Autodesk Inventor part; units mm, degrees
ref_plane "YZ Plane" through (0, 0, 0) normal (1, 0, 0) x (0, 1, 0)
ref_plane "XZ Plane" through (0, 0, 0) normal (0, 1, 0) x (-1, 0, 0)
ref_plane "XY Plane" through (0, 0, 0) normal (0, 0, 1) x (1, 0, 0)
sketch "Sketch1" plane through (0, 0, 0) normal (0, 1, 0) x (-1, 0, 0)
  line L0 (84.709, 4.7625) -> (-84.709, 4.7625)
  line L1 (-84.709, 4.7625) -> (-84.709, -4.7625)
  line L2 (-84.709, -4.7625) -> (84.709, -4.7625)
  line L3 (84.709, -4.7625) -> (84.709, 4.7625)
  line L4 (4.7625, 62.5475) -> (-4.7625, 62.5475)
  line L5 (-4.7625, 62.5475) -> (-4.7625, -91.4781)
  line L6 (-4.7625, -91.4781) -> (4.7625, -91.4781)
  line L7 (4.7625, -91.4781) -> (4.7625, 62.5475)
  point P0 (0, 0)
  point P1 (0, -4.7625)
  point P2 (84.709, 0)
  point P3 (4.7625, -14.4653)
  point P4 (0, 62.5475)
  dimension "d0" = 9.525
  dimension "d1" = 169.418
  dimension "d2" = 154.0256
  dimension "d6" = 57.785
extrude "Extrusion1" add sketch "Sketch1" along normal blind 6.35
sketch "Sketch2" plane through (0, 6.35, 0) normal (0, 1, 0) x (1, 0, 0)
  line L0 (4.7625, 91.4781) -> (-4.7625, 91.4781)
  line L1 (84.709, -4.7625) -> (84.709, 4.7625)
  line L2 (-4.7625, -62.5475) -> (4.7625, -62.5475)
  line L3 (-84.709, 4.7625) -> (-84.709, -4.7625)
  point P0 (0, 0)
  point P1 (0, 86.7791)
  point P2 (0, -57.8485)
  point P3 (-80.01, 0)
  point P4 (80.01, 0)
  dimension "d7" = 4.699
  dimension "d8" = 4.699
  dimension "d9" = 4.699
  dimension "d10" = 4.699
hole "Hole1" at (0, 6.35, -86.7791) at (0, 6.35, 57.8485) at (-80.01, 6.35, 0) at (80.01, 6.35, 0) direction (0, -1, 0) diameter 3.302 end through all
fillet "Fillet1" radius 1.27 20 edges at (-44.7358, 6.35, 4.7625) (4.7625, 6.35, 33.655) (-4.7625, 6.35, 33.655) (44.7357, 6.35, 4.7625) (4.7625, 6.35, -48.1203) (-4.7625, 6.35, -48.1203) (-44.7357, 6.35, -4.7625) (44.7358, 6.35, -4.7625) (84.709, 3.175, 4.7625) (84.709, 3.175, -4.7625) (84.709, 6.35, 0) (4.7625, 3.175, 62.5475) (0, 6.35, 62.5475) (-4.7625, 3.175, 62.5475) (-84.709, 3.175, 4.7625) (-84.709, 6.35, 0) (4.7625, 3.175, -91.4781) (0, 6.35, -91.4781) (-4.7625, 3.175, -91.4781) (-84.709, 3.175, -4.7625)
fillet "Fillet2" radius 1.27 8 edges at (4.3905, 5.978, 4.3905) (4.7625, 2.54, 4.7625) (4.3905, 5.978, -4.3905) (4.7625, 2.54, -4.7625) (-4.3905, 5.978, -4.3905) (-4.7625, 2.54, -4.7625) (-4.3905, 5.978, 4.3905) (-4.7625, 2.54, 4.7625)
properties part number "BatteryCrossStrap"
Here's how the part is built. I have some questions about the finished solid (model axes, mm). A direction names the side the tool comes from. Round coordinates to 2 decimals unless told otherwise and drop trailing zeros. Write each loop counter-clockwise with the first axis right and the second up, starting at its lowest first coordinate (ties: lowest second). Pieces come first, ordered by that corner, then holes.
1. Suppose I cut it at C-C (z = 29). List the corners of the cut face in (x, y) for me, and give its area (3 significant figures).
2. Suppose I cut it at A-A (y = 3). List the corners of the cut face in (x, z) for me.
3. Will these pins go through, and if not, where does the flat tip stop? pin 1 Ø1.5 at (y, z) = (2, 25.5) entering from -X; pin 2 Ø3 at (x, y) = (-28.5, 2) entering from +Z; pin 3 Ø1.5 at (y, z) = (3, -28.5) entering from +X.
4. For faces 1 (the flat face through (-4.762, 3, -49)), 2 (the flat face through (44, 3, 4.762)), 3 (the flat face through (-4.762, 3, 33)), which set-ups out of +Z, -Z, +X, -X, +Y, -Y let a thin tool reach every point of the face, with its end or its side?
5. I need wall thicknesses on L1, parallel to X at y = 2, z = 0; L2, parallel to Z at x = -80.01, y = 4.5; L3, parallel to X at y = 4.75, z = 12. Which ranges of each line are inside material? Lowest first, please.
6. Suppose I cut it at B-B (x = -55.5). List the corners of the cut face in (y, z) for me.
Answer sheet:
1. outline: (-4.76, 0) - (4.76, 0) - (4.76, 5.08) arc R1.27 ccw to (3.49, 6.35) - (-3.49, 6.35) arc R1.27 ccw to (-4.76, 5.08) - close
1. area: 59.8 mm2
2. outline: (-84.71, -3.49) arc R1.27 ccw to (-83.44, -4.76) - (-6.03, -4.76) arc R1.27 cw to (-4.76, -6.03) - (-4.76, -90.21) arc R1.27 ccw to (-3.49, -91.48) - (3.49, -91.48) arc R1.27 ccw to (4.76, -90.21) - (4.76, -6.03) arc R1.27 cw to (6.03, -4.76) - (83.44, -4.76) arc R1.27 ccw to (84.71, -3.49) - (84.71, 3.49) arc R1.27 ccw to (83.44, 4.76) - (6.03, 4.76) arc R1.27 cw to (4.76, 6.03) - (4.76, 61.28) arc R1.27 ccw to (3.49, 62.55) - (-3.49, 62.55) arc R1.27 ccw to (-4.76, 61.28) - (-4.76, 6.03) arc R1.27 cw to (-6.03, 4.76) - (-83.44, 4.76) arc R1.27 ccw to (-84.71, 3.49) - close; hole circle Ø3.3 at (-80.01, 0); hole circle Ø3.3 at (0, -86.78); hole circle Ø3.3 at (0, 57.85); hole circle Ø3.3 at (80.01, 0)
3. pin 1: stops at x = -4.76
3. pin 2: stops at z = 4.76
3. pin 3: stops at x = 4.76
4. face 1: -Z, -X, +Y, -Y
4. face 2: +Z, +X, +Y, -Y
4. face 3: +Z, -X, +Y, -Y
5. L1: x = -84.71 to -81.66, -78.36 to 78.36, 81.66 to 84.71
5. L2: z = -4.76 to -1.65, 1.65 to 4.76
5. L3: x = -4.76 to 4.76
6. outline: (0, -4.76) - (5.08, -4.76) arc R1.27 ccw to (6.35, -3.49) - (6.35, 3.49) arc R1.27 ccw to (5.08, 4.76) - (0, 4.76) - close
